```python
from build123d import *

# Parameters (mm, degrees)
F1_DEPTH = 20
F2_R     = 9.75
F3_DEPTH = 10


with BuildPart() as f1:
    # F0 (on Top) → F1 (new body)
    with BuildSketch(Plane.XY):
        with BuildLine():
            ThreePointArc((37.3205080757, 10), (39.3185165258, 14.8236190979), (40, 20))
            ThreePointArc((40, 20), (39.3185165258, 25.1763809021), (37.3205080757, 30))
            Line((37.3205080757, 30), (20, 30))
            Line((20, 30), (20, 10))
            Line((20, 10), (37.3205080757, 10))
        make_face()
        with BuildLine():
            ThreePointArc((37.3205080757, 30), (39.3185165258, 25.1763809021), (40, 20))
            ThreePointArc((40, 20), (39.3185165258, 14.8236190979), (37.3205080757, 10))
            Line((37.3205080757, 10), (44, 10))
            Line((44, 10), (44, 30))
            Line((44, 30), (37.3205080757, 30))
        make_face()
        with BuildLine():
            Line((20, 30), (37.3205080757, 30))
            ThreePointArc((37.3205080757, 30), (0, 20), (37.3205080757, 10))
            Line((37.3205080757, 10), (20, 10))
            Line((20, 10), (20, 30))
        make_face()
    extrude(amount=F1_DEPTH)

    # F2 (on face) → F3 (join)
    with BuildSketch(Plane.XY.offset(20)):
        with Locations((20, 20)):
            Circle(F2_R)
    extrude(amount=F3_DEPTH)


solid = f1.part
```
Part model, mm, in its own coordinate system. A direction names the side the tool comes from. Give positions to 0.01 mm unless a question says otherwise; leave off trailing zeros. Order: outer loops, then holes, each group sorted by start corner. A loop starts at its lowest first (then second) coordinate and runs counter-clockwise, first axis right, second up. Notation, with made-up numbers: M 22.5,67.25 L 58.5,67.25 A23 ccw 58.5,76.25 Z; hole C 18,-15.75 d4. An arc over 180 degrees is marked long. Use a Markdown table: item, result. Add a question column.
(1) Saw through at B-B, the plane y = 20. Give the cut face in (x, z).
(2) Probe line 1 along Z through (x, y) = (6.5, 29.5); line 2 along Y through (x, z) = (38, 10.5); line 3 along X through (y, z) = (19, 18.5). List the from-to ranges inside material, lowest first. Write a range as [from, to].
(3) Drop flat-ended pins along their axis: P1, Ø1, axis at x = 15.5, z = 15.5, coming from the -Y side; P2, Ø5.5, axis at x = 41, z = 13.5, coming from the +Y side; P3, Ø1, axis at y = 15, z = 19.5, coming from the -X side; P4, Ø1, axis at y = 32, z = 23, coming from the -X side. Give the stop position or say it passes through.
(4) 3-axis set-ups, long thin cutter, end or side, ignore diameter. For faces 1 (the face through (0.013, 20.733, 9.86)), 2 (the face through (12.26, 14.07, 24.93)), 3 (the face through (41, 10, 10)): which of +Z, -Z, +X, -X, +Y, -Y reach the whole face in a straight line?
(5) Saw through at D-D, the plane x = 4. Give the cut face in (y, z).
(6) Saw through at C-C, the plane z = 24.75. Give the cut face in (x, y).
(7) Saw through at A-A, the plane x = 20. Give the cut face in (y, z).
(8) Mould opens along Z. For faces 4 (the face through (20, 20, 30)), 5 (the face through (22, 20, 0)), 6 (the face through (41, 30, 10)) say: +Z half, -Z half, draft (parallel to the pull), parting line (faces both ways), or undercut.
Answer key:
| question | item | result |
|---|---|---|
| 1 | outline | M 0,0 L 44,0 L 44,20 L 29.75,20 L 29.75,30 L 10.25,30 L 10.25,20 L 0,20 Z |
| 2 | line 1 | [0, 20] |
| 2 | line 2 | [10, 30] |
| 2 | line 3 | [0.03, 44] |
| 3 | P1 | y = 0.4 |
| 3 | P2 | y = 30 |
| 3 | P3 | x = 0.51 |
| 3 | P4 | through |
| 4 | face 1 | +Z, -Z |
| 4 | face 2 | +Z |
| 4 | face 3 | +Z, -Z, +X, -Y |
| 5 | outline | M 8,0 L 32,0 L 32,20 L 8,20 Z |
| 6 | outline | C 20,20 d19.5 |
| 7 | outline | M 0,0 L 40,0 L 40,20 L 29.75,20 L 29.75,30 L 10.25,30 L 10.25,20 L 0,20 Z |
| 8 | face 4 | +Z half |
| 8 | face 5 | -Z half |
| 8 | face 6 | draft |
